Build history of the part. All positions in model axes, mm. A direction names the side the tool comes from. Give positions to 0.01 mm unless a question says otherwise; leave off trailing zeros. Order: outer loops, then holes, each group sorted by start corner. A loop starts at its lowest first (then second) coordinate and runs counter-clockwise, first axis right, second up. Notation, with made-up numbers: M -2,68.5 L 21,68.5 A11 ccw 21,80.5 Z; hole C -9,71.25 d6. An arc over 180 degrees is marked long. Use CSV: the item, a comma, the result in double quotes. Start each with the question number.
Item 1: Pin check, flat tips, straight feed: P1, Ø0.8, axis at y = 23.5, z = -4.5, coming from the -X side; P2, Ø0.8, axis at x = -14, y = 10, coming from the +Z side; P3, Ø0.8, axis at y = 9.5, z = -5, coming from the +X side. Stop position of each tip, or through.
Item 2: Band-saw the part on B-B on y = 7.5. Write the cut outline in (x, z), plus the area to 3 significant figures.
Item 3: Band-saw the part on C-C on z = 7.5. Write the cut outline in (x, y), plus the area to 4 significant figures.
Item 4: Which spindle directions (+Z, -Z, +X, -X, +Y, -Y) get a long thin tool onto all of the face, cutting with end or side? Do faces 5 (the cylindrical face through (7.451, 22.133, -31.948)), 6 (the cylindrical face through (-15.53, 11.18, -3.94)), 7 (the cylindrical face through (-12.529, 22.258, 13.7)), 8 (the cylindrical face through (10.1, 11.2, -24.9)). Say none if no direction does.
Item 5: Band-saw the part on D-D on y = 14. Write the cut outline in (x, z).
Item 6: Wall check: line 1 along X through (y, z) = (21, 1.5); line 2 along Z through (x, y) = (9.5, 23); line 3 along Z through (x, y) = (3, 20). Give the ranges that are in metal, low to high.
Item 7: Two-plate mould, pull along Y, no slides. Class faces 1 (the flat face through (-13, 28.1, -26)), 2 (the flat face through (-17.21, 16, -9)), 3 (the cylindrical face through (-11.845, 10.421, 13.7)), 4 (the flat face through (-13, 24, 11.976)): pulls with the +Y half, pulls with the -Y half, needs draft (parallel to the pull), parting line crosses it, or undercut.
Item 8: Band-saw the part on A-A on x = 5.5. Write the cut outline in (y, z), plus the area to 3 significant figures.
from build123d import *

# Parameters (mm, degrees)
SKETCH1_W           = 29
SKETCH1_H           = 49
BOSS_EXTRUDE1_DEPTH = 31.5
SKETCH2_W           = 18
SKETCH2_H           = 10
CUT_EXTRUDE1_DEPTH  = 32.5
SKETCH3_R           = 1.4
CUT_EXTRUDE2_DEPTH  = 3.4
SKETCH4_R           = 1.4
CUT_EXTRUDE3_DEPTH  = 3.4
SKETCH5_R           = 1.4
CUT_EXTRUDE4_DEPTH  = 3.4
CUT_EXTRUDE5_DEPTH  = 12


with BuildPart() as part:
    # Sketch1 → Boss-Extrude1 (new body)
    with BuildSketch(Plane(origin=(0, 0, 0), x_dir=(1, 0, 0), z_dir=(0, 1, 0))):
        with Locations((-2.710031348, 9.123824451)):
            Rectangle(SKETCH1_W, SKETCH1_H)
    extrude(amount=BOSS_EXTRUDE1_DEPTH)

    # Sketch2 → Cut-Extrude1 (cut, through all)
    with BuildSketch(Plane(origin=(0, 31.5, 0), x_dir=(1, 0, 0), z_dir=(0, 1, 0))):
        with Locations((-2.710031348, -4.376175549)):
            Rectangle(SKETCH2_W, SKETCH2_H)
    extrude(amount=-CUT_EXTRUDE1_DEPTH, mode=Mode.SUBTRACT)

    # Sketch3 → Cut-Extrude2 (cut)
    with BuildSketch(Plane(origin=(0, 31.5, 0), x_dir=(1, 0, 0), z_dir=(0, 1, 0))):
        with Locations((-13.175031348, 25.623824451)):
            Circle(SKETCH3_R)
        with Locations((-13.175031348, 12.123824451)):
            Circle(SKETCH3_R)
        with Locations((7.754968652, 25.623824451)):
            Circle(SKETCH3_R)
        with Locations((7.754968652, 12.123824451)):
            Circle(SKETCH3_R)
    extrude(amount=-CUT_EXTRUDE2_DEPTH, mode=Mode.SUBTRACT)

    # Sketch4 → Cut-Extrude3 (cut)
    with BuildSketch(Plane.ZY.offset(17.210031348)):
        with Locations((-25.623824451, 23.5)):
            Circle(SKETCH4_R)
        with Locations((-4.693824451, 23.5)):
            Circle(SKETCH4_R)
        with Locations((-25.623824451, 10)):
            Circle(SKETCH4_R)
        with Locations((-4.693824451, 10)):
            Circle(SKETCH4_R)
    cut_extrude3 = extrude(amount=-CUT_EXTRUDE3_DEPTH, mode=Mode.SUBTRACT)

    # Mirror1: Cut-Extrude3 across plane
    add(cut_extrude3.mirror(Plane.ZY.offset(2.710031348)), mode=Mode.SUBTRACT)

    # Sketch5 → Cut-Extrude4 (cut)
    with BuildSketch(Plane.XY.offset(15.376175549)):
        with Locations((-13.175031348, 23.5)):
            Circle(SKETCH5_R)
        with Locations((7.754968652, 23.5)):
            Circle(SKETCH5_R)
        with Locations((-13.180031348, 10)):
            Circle(SKETCH5_R)
        with Locations((7.749968652, 10)):
            Circle(SKETCH5_R)
    cut_extrude4 = extrude(amount=-CUT_EXTRUDE4_DEPTH, mode=Mode.SUBTRACT)

    # Mirror2: Cut-Extrude4 across plane
    add(cut_extrude4.mirror(Plane.XY.offset(-9.123824451)), mode=Mode.SUBTRACT)

    # Sketch7 → Cut-Extrude5 (cut)
    with BuildSketch(Plane.XZ):
        Polygon((3.929496748, -17.123824451), (0.6097327, -11.373824451), (-6.029795396, -11.373824451), (-9.349559444, -17.123824451), (-6.029795396, -22.873824451), (0.6097327, -22.873824451), align=None)
    extrude(amount=-CUT_EXTRUDE5_DEPTH, mode=Mode.SUBTRACT)


solid = part.part
Model answer:
1,P1,"stops at x = -13.81"
1,P2,"stops at z = 11.98"
1,P3,"stops at x = 8.39"
2,outline,"M -17.21,-33.62 L 11.79,-33.62 L 11.79,15.38 L -17.21,15.38 Z; hole M -11.71,-0.62 L 6.29,-0.62 L 6.29,9.38 L -11.71,9.38 Z; hole M -9.35,-17.12 L -6.03,-22.87 L 0.61,-22.87 L 3.93,-17.12 L 0.61,-11.37 L -6.03,-11.37 Z"
2,area,"1,130 mm^2"
3,outline,"M -17.21,0 L -11.71,0 L -11.71,31.5 L -17.21,31.5 Z; M 6.29,0 L 11.79,0 L 11.79,31.5 L 6.29,31.5 Z"
3,area,"346.5 mm^2"
4,face 5,"-Z"
4,face 6,"-X"
4,face 7,"+Z"
4,face 8,"+X"
5,outline,"M -17.21,-33.62 L 11.79,-33.62 L 11.79,15.38 L -17.21,15.38 Z; hole M -11.71,-0.62 L 6.29,-0.62 L 6.29,9.38 L -11.71,9.38 Z"
6,line 1,"x = -17.21 to -11.71, 6.29 to 11.79"
6,line 2,"z = -33.62 to -26.93, -24.32 to -6, -3.39 to 15.38"
6,line 3,"z = -33.62 to -0.62, 9.38 to 15.38"
7,face 1,"pulls with the +Y half"
7,face 2,"needs draft"
7,face 3,"undercut"
7,face 4,"undercut"
8,outline,"M 0,-33.62 L 31.5,-33.62 L 31.5,-0.62 L 0,-0.62 Z; M 0,9.38 L 31.5,9.38 L 31.5,15.38 L 0,15.38 Z"
8,area,"1,230 mm^2"
